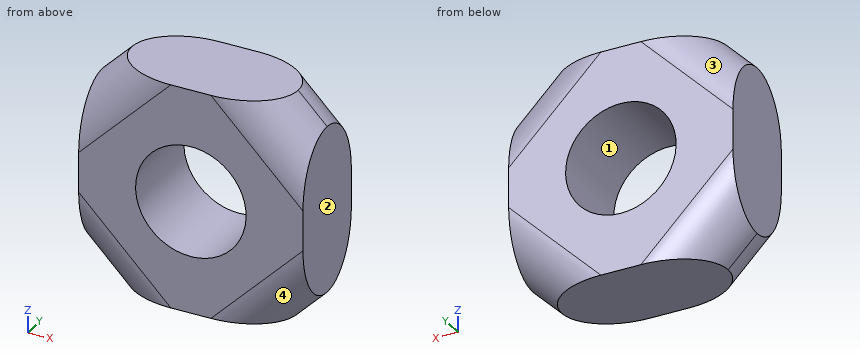
```python
from build123d import *

# Parameters (mm, degrees)
EXTRUDE_1_DEPTH        = 5.5
FILLET_1_R             = 2.75
HOLE_WIZARD_M8_1_D     = 6.8
HOLE_WIZARD_M8_1_DEPTH = 19.75
HOLE_WIZARD_M8_1_TIP   = 2.042926105


with BuildPart() as part:
    # 草图1 → 凸台-拉伸1 (new body)
    with BuildSketch(Plane(origin=(0, 0, 0), x_dir=(1, 0, 0), z_dir=(0, 1, 0))):
        Polygon((0, 0), (10.24163056, 0), (12.02081528, 1.77918472), (12.02081528, 12.02081528), (10.24163056, 13.8), (0, 13.8), (-1.77918472, 12.02081528), (-1.77918472, 1.77918472), align=None)
    extrude(amount=EXTRUDE_1_DEPTH)

    # 圆角1
    fillet_1_edges = [part.edges().sort_by_distance(p)[0] for p in [
        (-0.88959236, 0, -12.91040764),
        (-0.88959236, 5.5, -12.91040764),
        (11.13122292, 0, -12.91040764),
        (11.13122292, 5.5, -12.91040764),
        (11.13122292, 0, -0.88959236),
        (11.13122292, 5.5, -0.88959236),
        (-0.88959236, 0, -0.88959236),
        (-0.88959236, 5.5, -0.88959236),
    ]]
    fillet(fillet_1_edges, radius=FILLET_1_R - 0.0001)  # a hair under: the kernel refuses the full size

    # M8 螺纹孔1
    with Locations(Plane(origin=(5.12081528, 5.5, -6.9), x_dir=(0, 0, 1), z_dir=(0, 1, 0))):
        with Locations((0, 0)):
            Hole(HOLE_WIZARD_M8_1_D / 2, depth=HOLE_WIZARD_M8_1_DEPTH)
            with Locations((0, 0, -(HOLE_WIZARD_M8_1_DEPTH + HOLE_WIZARD_M8_1_TIP / 2))):  # 118° drill point
                Cone(0, HOLE_WIZARD_M8_1_D / 2, HOLE_WIZARD_M8_1_TIP, mode=Mode.SUBTRACT)


solid = part.part
```
Geometry: final body of the model. Coordinates: model frame, mm. Face numbers are marked on the shaded views. Round coordinates to 2 decimals unless told otherwise and drop trailing zeros. Write each loop counter-clockwise with the first axis right and the second up, starting at its lowest first coordinate (ties: lowest second). Pieces come first, ordered by that corner, then holes.
Item 1: Pin query (flat end, axial travel): P1, Ø1, axis at x = 4, z = -9.5, coming from the -Y side (1 decimal). Return the tip coordinate at first contact, or that it passes through.
Item 2: Section query B-B (y = 3.3). Return loops of the section in (x, z), plus the area to 3 significant figures.
Item 3: Section query A-A (z = -6.9). Return loops of the section in (x, y).
Item 4: Mould query, pull axis Z, two halves, no side actions, for the marked faces 1, 2, 3 and 4. Classes: +Z half, -Z half, draft (parallel to the pull), parting line (faces both ways), or undercut.
Item 5: Section query C-C (y = 4.5). Return loops of the section in (x, z), plus the area to 3 significant figures.
Item 6: Material intervals for L1, parallel to X at y = 3.6, z = -6.9; L2, parallel to X at y = 4.35, z = -9; L3, parallel to Z at x = 8, y = 1, sorted ascending.
Completed:
1. P1: passes through
2. outline: (-1.78, -11.94) - (0.08, -13.8) - (10.16, -13.8) - (12.02, -11.94) - (12.02, -1.86) - (10.16, 0) - (0.08, 0) - (-1.78, -1.86) - close; hole circle Ø6.8 at (5.12, -6.9)
2. area: 147 mm2
3. outline: (-1.78, 0) - (1.72, 0) - (1.72, 5.5) - (-1.78, 5.5) - close; (8.52, 0) - (12.02, 0) - (12.02, 5.5) - (8.52, 5.5) - close
4. face 1: undercut
4. face 2: draft
4. face 3: +Z half
4. face 4: -Z half
5. outline: (-1.78, -11.13) - (0.89, -13.8) - (9.35, -13.8) - (12.02, -11.13) - (12.02, -2.67) - (9.35, 0) - (0.89, 0) - (-1.78, -2.67) - close; hole circle Ø6.8 at (5.12, -6.9)
5. area: 140 mm2
6. L1: x = -1.78 to 1.72, 8.52 to 12.02
6. L2: x = -1.78 to 2.45, 7.79 to 12.02
6. L3: z = -13.8 to -8.71, -5.09 to 0
